Geometry: final body of the model. Coordinates: model frame, mm. Give positions to 0.01 mm unless a question says otherwise; leave off trailing zeros. Write each loop counter-clockwise with the first axis right and the second up, starting at its lowest first coordinate (ties: lowest second). Pieces come first, ordered by that corner, then holes. Notation, with made-up numbers: (8, -6.75) -> (14, -6.75) arc R26 cw to (14, 11.25) -> close; hole circle Ø6 at (-20.75, -14). An arc over 180 degrees is marked (long way). Answer in a Markdown table with one row per item. Add a question column.
Item 1: Section query A-A on z = 30. Output: boundary loops of the cut face in (x, y), plus the area to 3 significant figures.
Item 2: Section query B-B on x = 25.5. Output: boundary loops of the cut face in (y, z).
Item 3: Material intervals for probe 1 along Z at (x, y) = (-4.5, -34.45); probe 2 along Z at (x, y) = (65.5, -32.8); probe 3 along X at (y, z) = (-34.75, 70), sorted ascending. Write a range as from..to.
Item 4: Section query D-D on y = -33.9. State how many separate pieces and enclosed holes the cut face has, plus the area to 3 significant figures.
Item 5: Section query C-C on z = 4.5. Output: boundary loops of the cut face in (x, y), plus the area to 3 significant figures.
Item 6: First-contact query: P1, Ø4, axis at x = 65.5, z = 20, coming from the -Y side. Flat tip, straight axial feed; report the tip coordinate or a pass-through.
```python
from build123d import *

# Parameters (mm, degrees)
CYLINDER038_R            = 1.8
CYLINDER038_DEPTH        = 100
ARRAY001_X_COUNT         = 2
ARRAY001_X_PITCH         = 25
ARRAY001_Y_COUNT         = 2
ARRAY001_Y_PITCH         = 11
ARRAY001_PLACEMENT_ANGLE = 90
ARRAY002_Z_COUNT         = 2
ARRAY002_Z_PITCH         = 80
CYLINDER011003_R         = 1.8
CYLINDER011003_DEPTH     = 10
ARRAY005_X_COUNT         = 2
ARRAY005_X_PITCH         = 30
ARRAY005_Y_COUNT         = 2
ARRAY005_Y_PITCH         = 20
ARRAY005_PITCH_ANGLE     = 90
ARRAY005_PLACEMENT_ANGLE = -90
BOX002_W                 = 22
BOX002_H                 = 10
BOX002_DEPTH             = 50
FILLET002_R              = 3
BOX003_W                 = 16
BOX003_H                 = 200
BOX003_DEPTH             = 50
CYLINDER_R               = 8
CYLINDER_DEPTH           = 200
SKETCH_W                 = 42.117567
SKETCH_H                 = 23.738708
SKETCH_W_2               = 40.471139
SKETCH_H_2               = 27.047569
SKETCH_W_3               = 29.381024
SKETCH_H_3               = 46.19655
SKETCH_W_4               = 20.234924
SKETCH_H_4               = 18.049118
SKETCH_W_5               = 22.001269
SKETCH_H_5               = 17.778789
SKETCH_W_6               = 9.111635
SKETCH_H_6               = 47.113838
EXTRUDE_DEPTH            = 50
CYLINDER011002_R         = 1.8
CYLINDER011002_DEPTH     = 100
ARRAY004_X_COUNT         = 9
ARRAY004_X_PITCH         = 10
ARRAY004_Z_COUNT         = 9
ARRAY004_Z_PITCH         = 10
BOX_W                    = 97
BOX_H                    = 5
BOX_DEPTH                = 100
FILLET_R                 = 2


with BuildPart() as bolt_hole_array_pair:
    # Cylinder038 → Cylinder038 (new body)
    with BuildSketch(Plane.XY.offset(-50)):
        Circle(CYLINDER038_R)
    extrude(amount=CYLINDER038_DEPTH)

    # Array001 X: bolt hole array pair ×2


with BuildPart() as bolt_hole_array_pair_1:
    add(bolt_hole_array_pair.part)
    with Locations(*[(i * ARRAY001_X_PITCH, 0, 0) for i in range(1, ARRAY001_X_COUNT)]):
        add(bolt_hole_array_pair.part)

    # Array001 Y: bolt hole array pair ×2


with BuildPart() as bolt_hole_array_pair_2:
    add(bolt_hole_array_pair_1.part)
    with Locations(*[(0, i * ARRAY001_Y_PITCH, 0) for i in range(1, ARRAY001_Y_COUNT)]):
        add(bolt_hole_array_pair_1.part)


with BuildPart() as bolt_hole_array_pair_3:
    # Array001 placement: moved
    add(bolt_hole_array_pair_2.part.moved(Location((-12.5, 0, 4.5))).rotate(Axis((-12.5, 0, 4.5), (1, 0, 0)), ARRAY001_PLACEMENT_ANGLE))

    # Array002 Z: bolt hole array pair ×2


with BuildPart() as bolt_hole_array_pair_4:
    add(bolt_hole_array_pair_3.part)
    with Locations(*[(0, 0, i * ARRAY002_Z_PITCH) for i in range(1, ARRAY002_Z_COUNT)]):
        add(bolt_hole_array_pair_3.part)


with BuildPart() as stepper_mount_hole_array:
    # Cylinder011003 → Cylinder011003 (new body)
    with BuildSketch(Plane.XY):
        Circle(CYLINDER011003_R)
    extrude(amount=CYLINDER011003_DEPTH)

    # Array005 X: stepper mount hole array ×2


with BuildPart() as stepper_mount_hole_array_1:
    add(stepper_mount_hole_array.part)
    with Locations(*[(i * ARRAY005_X_PITCH, 0, 0) for i in range(1, ARRAY005_X_COUNT)]):
        add(stepper_mount_hole_array.part)

    # Array005 Y: stepper mount hole array ×2


with BuildPart() as stepper_mount_hole_array_2:
    add(stepper_mount_hole_array_1.part)
    with Locations(*[(0, i * ARRAY005_Y_PITCH, 0) for i in range(1, ARRAY005_Y_COUNT)]):
        add(stepper_mount_hole_array_1.part)


with BuildPart() as stepper_mount_hole_array_3:
    # Array005 pitch: moved
    add(stepper_mount_hole_array_2.part.rotate(Axis((0, 0, 0), (0, 1, 0)), ARRAY005_PITCH_ANGLE))


with BuildPart() as stepper_mount_hole_array_4:
    # Array005 placement: moved
    add(stepper_mount_hole_array_3.part.moved(Location((48, -31, 65))).rotate(Axis((48, -31, 65), (0, 0, 1)), ARRAY005_PLACEMENT_ANGLE))


with BuildPart() as belt_hole_fillet:
    # Box002 → Box002 (new body)
    with BuildSketch(Plane(origin=(18, -40, 25), x_dir=(1, 0, 0), z_dir=(0, 0, 1))):
        with Locations((11, 5)):
            Rectangle(BOX002_W, BOX002_H)
    extrude(amount=BOX002_DEPTH)

    # Fillet002
    fillet002_edges = [belt_hole_fillet.edges().sort_by_distance(p)[0] for p in [
        (18, -35, 75),
        (18, -35, 25),
        (40, -35, 75),
        (40, -35, 25),
    ]]
    fillet(fillet002_edges, radius=FILLET002_R)


with BuildPart() as shaft_extension_cube:
    # Box003 → Box003 (new body)
    with BuildSketch(Plane(origin=(-8, -200, -50), x_dir=(1, 0, 0), z_dir=(0, 0, 1))):
        with Locations((8, 100)):
            Rectangle(BOX003_W, BOX003_H)
    extrude(amount=BOX003_DEPTH)


with BuildPart() as shaft_16mm_hole:
    # Cylinder → Cylinder (new body)
    with BuildSketch(Plane.XZ):
        Circle(CYLINDER_R)
    extrude(amount=CYLINDER_DEPTH)

    # Fusion002: union shaft extension cube
    add(shaft_extension_cube.part)


with BuildPart() as shaft_16mm_hole_1:
    # Fusion002 placement: moved
    add(shaft_16mm_hole.part.moved(Location((40, -19, 0))))


with BuildPart() as part_mirroring:
    # Part__Mirroring: instance of shaft 16mm hole
    add(shaft_16mm_hole_1.part.mirror(Plane(origin=(0, 0, 50), x_dir=(0, 1, 0), z_dir=(0, 0, 1))))


with BuildPart() as general_holes_extrude:
    # Sketch → Extrude (new body, symmetric)
    with BuildSketch(Plane.XZ):
        with Locations((-1.795196, 11.674214)):
            Rectangle(SKETCH_W, SKETCH_H)
        with Locations((-0.985158, 89.151065)):
            Rectangle(SKETCH_W_2, SKETCH_H_2)
        with Locations((57.017252, 49.302802)):
            Rectangle(SKETCH_W_3, SKETCH_H_3)
        with Locations((41.531349, 93.530205)):
            Rectangle(SKETCH_W_4, SKETCH_H_4)
        with Locations((39.547934, 5.882593)):
            Rectangle(SKETCH_W_5, SKETCH_H_5)
        with Locations((15.74623, 50.03809)):
            Rectangle(SKETCH_W_6, SKETCH_H_6)
    extrude(amount=EXTRUDE_DEPTH, both=True)


with BuildPart() as hole_fusion:
    # Cylinder011002 → Cylinder011002 (new body)
    with BuildSketch(Plane.XZ.offset(-50)):
        Circle(CYLINDER011002_R)
    extrude(amount=CYLINDER011002_DEPTH)

    # Array004 X: hole fusion ×9


with BuildPart() as hole_fusion_1:
    add(hole_fusion.part)
    with Locations(*[(i * ARRAY004_X_PITCH, 0, 0) for i in range(1, ARRAY004_X_COUNT)]):
        add(hole_fusion.part)

    # Array004 Z: hole fusion ×9


with BuildPart() as hole_fusion_2:
    add(hole_fusion_1.part)
    with Locations(*[(0, 0, i * ARRAY004_Z_PITCH) for i in range(1, ARRAY004_Z_COUNT)]):
        add(hole_fusion_1.part)


with BuildPart() as hole_fusion_3:
    # Array004 placement: moved
    add(hole_fusion_2.part.moved(Location((-14.5, 0, 10))))

    # Cut: cut general holes extrude
    add(general_holes_extrude.part, mode=Mode.SUBTRACT)

    # Fusion: union bolt hole array pair, stepper mount hole array, belt hole fillet, Part__Mirroring, shaft 16mm hole
    add(bolt_hole_array_pair_4.part)
    add(stepper_mount_hole_array_4.part)
    add(belt_hole_fillet.part)
    add(part_mirroring.part)
    add(shaft_16mm_hole_1.part)


with BuildPart() as side_plate_cut:
    # Box → Box (new body)
    with BuildSketch(Plane(origin=(-23, -36, 0), x_dir=(1, 0, 0), z_dir=(0, 0, 1))):
        with Locations((48.5, 2.5)):
            Rectangle(BOX_W, BOX_H)
    extrude(amount=BOX_DEPTH)

    # Fillet
    fillet_edges = [side_plate_cut.edges().sort_by_distance(p)[0] for p in [
        (-23, -33.5, 100),
        (-23, -33.5, 0),
        (74, -33.5, 100),
        (74, -33.5, 0),
    ]]
    fillet(fillet_edges, radius=FILLET_R)

    # Cut023015009002: cut hole fusion
    add(hole_fusion_3.part, mode=Mode.SUBTRACT)


solid = side_plate_cut.part
```
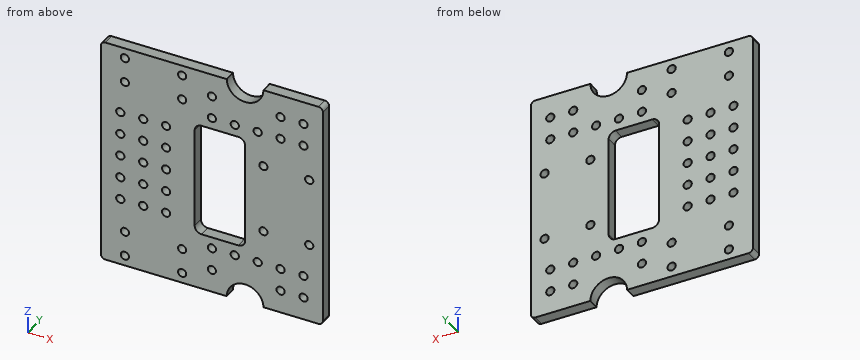
Findings below:
| question | item | result |
|---|---|---|
| 1 | outline | (-23, -36) -> (-16.3, -36) -> (-16.3, -31) -> (-23, -31) -> close; (-12.7, -36) -> (-6.3, -36) -> (-6.3, -31) -> (-12.7, -31) -> close; (-2.7, -36) -> (3.7, -36) -> (3.7, -31) -> (-2.7, -31) -> close; (7.3, -36) -> (18, -36) -> (18, -31) -> (7.3, -31) -> close; (40, -36) -> (74, -36) -> (74, -31) -> (40, -31) -> close |
| 1 | area | 321 mm^2 |
| 2 | outline | (-36, 0) -> (-31, 0) -> (-31, 8.2) -> (-36, 8.2) -> close; (-36, 11.8) -> (-31, 11.8) -> (-31, 18.2) -> (-36, 18.2) -> close; (-36, 21.8) -> (-31, 21.8) -> (-31, 25) -> (-36, 25) -> close; (-36, 75) -> (-31, 75) -> (-31, 78.2) -> (-36, 78.2) -> close; (-36, 81.8) -> (-31, 81.8) -> (-31, 88.2) -> (-36, 88.2) -> close; (-36, 91.8) -> (-31, 91.8) -> (-31, 100) -> (-36, 100) -> close |
| 3 | probe 1 | z = 0..28.2, 31.8..38.2, 41.8..48.2, 51.8..58.2, 61.8..68.2, 71.8..100 |
| 3 | probe 2 | z = 0..8.2, 11.8..18.2, 21.8..78.2, 81.8..88.2, 91.8..100 |
| 3 | probe 3 | x = -23..-16.3, -12.7..-6.3, -2.7..3.7, 7.3..18, 40..74 |
| 4 | separate pieces | 1 |
| 4 | enclosed holes | 44 |
| 4 | area | 7,970 mm^2 |
| 5 | outline | (-23, -36) -> (-14.3, -36) -> (-14.3, -31) -> (-23, -31) -> close; (-10.7, -36) -> (10.7, -36) -> (10.7, -31) -> (-10.7, -31) -> close; (14.3, -36) -> (33.39, -36) -> (33.39, -31) -> (14.3, -31) -> close; (46.61, -36) -> (74, -36) -> (74, -31) -> (46.61, -31) -> close |
| 5 | area | 383 mm^2 |
| 6 | P1 | stops at y = -36 |
